The drawing under review shows one solid part. Ordinate dimensions are in mm from its lowest x, y, z. A direction names the side the tool comes from. Round coordinates to 2 decimals unless told otherwise and drop trailing zeros. Order: outer loops, then holes, each group sorted by start corner. A loop starts at its lowest first (then second) coordinate and runs counter-clockwise, first axis right, second up.
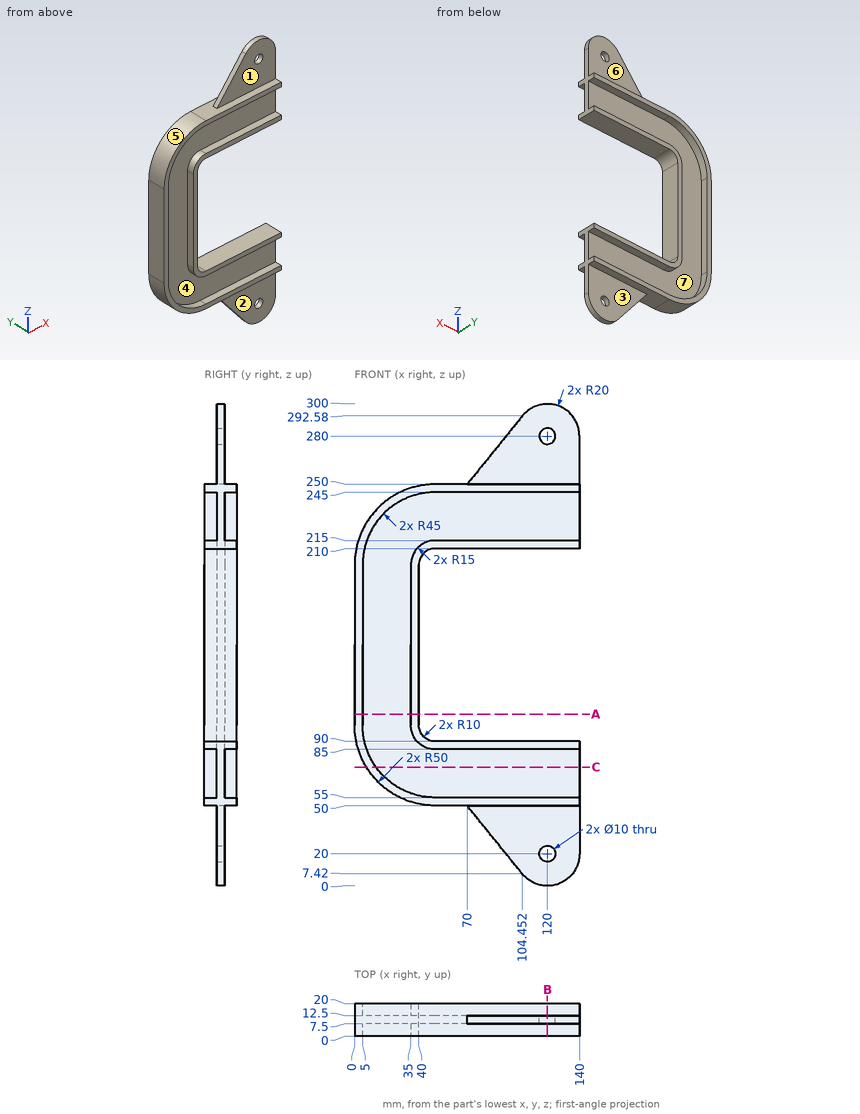
(1) To check wall thickness, follow L1, parallel to Z at x = 124.5, y = 1.5; L2, parallel to Z at x = 120, y = 8.65; L3, parallel to X at y = 16, z = 142. State the ranges of each line that lie inside material, in increasing order.
(2) Tool access review of the marked faces 1, 2 and 3: name each direction out of +Z, -Z, +X, -X, +Y, -Y from which nothing blocks a thin tool from reaching the whole face with its end or side.
(3) We need section A-A (z = 107). Give the boundary of the cut face in (x, y).
(4) We need section C-C (z = 74). Give the boundary of the cut face in (x, y).
(5) The part is to be moulded in two halves that separate along X. For the marked faces 4, 5, 6 and 7, say which applies: pulls with the +X half, pulls with the -X half, needs draft (parallel to the pull), parting line crosses it, or undercut.
(6) We need section B-B (x = 120). Count the separate pieces of the cut face and the enclosed holes in it, and give its area (3 significant figures).
(7) Clearance check with flat-ended pins moving along their axes: P1, Ø6, axis at x = 104.5, y = 5, coming from the +Z side; P2, Ø2, axis at x = 110, y = 17, coming from the -Z side; P3, Ø1, axis at x = 26, y = 16, coming from the +Z side; P4, Ø3, axis at x = 34, z = 118.5, coming from the -Y side. State where each tip first meets the part, or that it passes through.
Verdict:
1. L1: z = 50 to 55, 85 to 90, 210 to 215, 245 to 250
1. L2: z = 0 to 15, 25 to 90, 210 to 275, 285 to 300
1. L3: x = 0 to 5, 35 to 40
2. face 1: +Z, +X, -X, -Y
2. face 2: -Z, +X, -X, -Y
2. face 3: -Z, +X, -X, +Y
3. outline: (0, 0) - (5, 0) - (5, 7.5) - (35, 7.5) - (35, 0) - (40, 0) - (40, 20) - (35, 20) - (35, 12.5) - (5, 12.5) - (5, 20) - (0, 20) - close
4. outline: (7.29, 0) - (13.27, 0) - (13.27, 7.5) - (140, 7.5) - (140, 12.5) - (13.27, 12.5) - (13.27, 20) - (7.29, 20) - close
5. face 4: undercut
5. face 5: pulls with the -X half
5. face 6: needs draft
5. face 7: undercut
6. separate pieces: 4
6. enclosed holes: 0
6. area: 1,100 mm2
7. P1: stops at z = 294.44
7. P2: stops at z = 50
7. P3: stops at z = 244.13
7. P4: stops at y = 0
